Check sheet for the modelled part. Datum: model origin and axes. Units: mm. A direction names the side the tool comes from. Round coordinates to 2 decimals unless told otherwise and drop trailing zeros. Loops run counter-clockwise (first coordinate to the right, second up) from the corner with the lowest first, then second, coordinate; pieces in that order, holes last. Notation, with made-up numbers: (79.25, -18.75) - (87.25, -18.75) arc R17 cw to (87.25, -6.75) - close; hole circle Ø10 at (-22, 4). An arc over 180 degrees is marked (long way). Return JSON: item names as keys, results as strings.
from build123d import *

# Parameters (mm, degrees)
SKETCH1_R           = 23.5
BOSS_EXTRUDE1_DEPTH = 12
SKETCH2_R           = 16.75
BOSS_EXTRUDE2_DEPTH = 3.25
SKETCH3_R           = 10
CUT_EXTRUDE1_DEPTH  = 37.56586523
SKETCH5_R           = 20.75
SKETCH5_R_2         = 19.25
BOSS_EXTRUDE3_DEPTH = 2
FILLET1_R           = 1
FILLET2_R           = 1
FILLET3_R           = 0.5
FILLET4_R           = 0.5
SKETCH6_R           = 18.5
CUT_EXTRUDE2_DEPTH  = 0.5
FILLET5_R           = 0.5


with BuildPart() as part:
    # Sketch1 → Boss-Extrude1 (new body)
    with BuildSketch(Plane(origin=(0, 0, 0), x_dir=(1, 0, 0), z_dir=(0, 1, 0))):
        with Locations(Location((0, 0, 0), (0, 0, 270))):
            Circle(SKETCH1_R)
    extrude(amount=BOSS_EXTRUDE1_DEPTH)

    # Sketch2 → Boss-Extrude2 (add)
    with BuildSketch(Plane(origin=(0, 12, 0), x_dir=(1, 0, 0), z_dir=(0, 1, 0))):
        with Locations(Location((0, 0, 0), (0, 0, 90))):
            Circle(SKETCH2_R)
    extrude(amount=BOSS_EXTRUDE2_DEPTH)

    # Sketch3 → Cut-Extrude1 (cut, through all)
    with BuildSketch(Plane(origin=(0, 15.25, 0), x_dir=(1, 0, 0), z_dir=(0, 1, 0))):
        with Locations(Location((0, 0, 0), (0, 0, 270))):
            Circle(SKETCH3_R)
    extrude(amount=-CUT_EXTRUDE1_DEPTH, mode=Mode.SUBTRACT)

    # Sketch5 → Boss-Extrude3 (add)
    with BuildSketch(Plane(origin=(0, 12, 0), x_dir=(1, 0, 0), z_dir=(0, 1, 0))):
        with Locations(Location((0, 0, 0), (0, 0, 270))):
            Circle(SKETCH5_R)
        with Locations(Location((0, 0, 0), (0, 0, 270))):
            Circle(SKETCH5_R_2, mode=Mode.SUBTRACT)
    extrude(amount=BOSS_EXTRUDE3_DEPTH)

    # Fillet1
    fillet1_edges = [part.edges().sort_by_distance(p)[0] for p in [
        (0, 0, -23.5),
    ]]
    fillet(fillet1_edges, radius=FILLET1_R)

    # Fillet2
    fillet2_edges = [part.edges().sort_by_distance(p)[0] for p in [
        (0, 15.25, -10),
    ]]
    fillet(fillet2_edges, radius=FILLET2_R)

    # Fillet3
    fillet3_edges = [part.edges().sort_by_distance(p)[0] for p in [
        (0, 15.25, 16.75),
    ]]
    fillet(fillet3_edges, radius=FILLET3_R)

    # Fillet4
    fillet4_edges = [part.edges().sort_by_distance(p)[0] for p in [
        (0, 0, -10),
        (0, 12, -23.5),
    ]]
    fillet(fillet4_edges, radius=FILLET4_R)

    # Sketch6 → Cut-Extrude2 (cut)
    with BuildSketch(Plane(origin=(0, 0, 0), x_dir=(-1, 0, 0), z_dir=(0, -1, 0))):
        with Locations(Location((0, 0, 0), (0, 0, 90))):
            Circle(SKETCH6_R)
    extrude(amount=-CUT_EXTRUDE2_DEPTH, mode=Mode.SUBTRACT)

    # Fillet5
    fillet5_edges = [part.edges().sort_by_distance(p)[0] for p in [
        (0, 0.5, -10),
    ]]
    fillet(fillet5_edges, radius=FILLET5_R)


solid = part.part
Q1. Draft check along X on faces 4 (the face through (6.2, 13, 19.8)), 5 (the face through (-14, 14, 14)), 6 (the face through (-17, 12, -2)). Enter one of: released by +X, released by -X, zero draft, split by the parting line, or undercut.
Answer key:
{"face 4": "split by the parting line", "face 5": "zero draft", "face 6": "undercut"}
Q2. Depth check by flat-ended pin: P1, Ø2, axis at x = 0, z = 16, coming from the -Y side; P2, Ø18, axis at x = 0, z = 0, coming from the +Y side; P3, Ø3, axis at x = -13, y = 11.5, coming from the +Z side; P4, Ø4, axis at y = 3, z = 17, coming from the +X side. Enter the tip coordinate at first touch or a pass-through.
Answer key:
{"P1": "stops at y = 0.5", "P2": "passes through", "P3": "stops at z = 20.49", "P4": "stops at x = 18.09"}
Q3. Sectioned sample at B-B (y = 13). Enter the section's corners in (x, z).
Answer key:
{"outline": "circle Ø41.5 at (0, 0); circle Ø33.5 at (0, 0); hole circle Ø38.5 at (0, 0); hole circle Ø20 at (0, 0)"}
Q4. Scan lines: probe 1 along X at (y, z) = (13.35, 0); probe 2 along X at (y, z) = (9, 0); probe 3 along X at (y, z) = (14.75, 0). Record each from-to range of solid material in increasing order. Write a range as [from, to].
Answer key:
{"probe 1": "x = [-20.75, -19.25], [-16.75, -10], [10, 16.75], [19.25, 20.75]", "probe 2": "x = [-23.5, -10], [10, 23.5]", "probe 3": "x = [-16.75, -10.13], [10.13, 16.75]"}
Q5. Sectioned sample at D-D (y = 9.25). Enter the section's corners in (x, z), plus the area to 3 significant figures.
Answer key:
{"outline": "circle Ø47 at (0, 0); hole circle Ø20 at (0, 0)", "area": "1,420 mm²"}
Q6. Tool access check on faces 1 (the face through (-7.086, 0.246, -17.089)), 2 (the face through (-18, 0, -5)), 3 (the face through (14.86, 13.36, -7.73)). Record the directions out of +Z, -Z, +X, -X, +Y, -Y that give a thin tool (end or side, any length) a straight path to the whole face; none if there is none.
Answer key:
{"face 1": "-Y", "face 2": "+Z, -Z, +X, -X, -Y", "face 3": "+Y"}
